Geometry: see drawing. Coordinates: mm, zero at the bounding-box minimum. A direction names the side the tool comes from. Round coordinates to 2 decimals unless told otherwise and drop trailing zeros. Write each loop counter-clockwise with the first axis right and the second up, starting at its lowest first coordinate (ties: lowest second). Pieces come first, ordered by that corner, then holes. Notation, with made-up numbers: (-7.75, 24.5) -> (25.25, 24.5) arc R13 ccw to (25.25, 35.5) -> close; hole circle Ø3 at (77.5, -13). An arc over 180 degrees is marked (long way). Use CSV: the item, a comma, the result in double quotes.
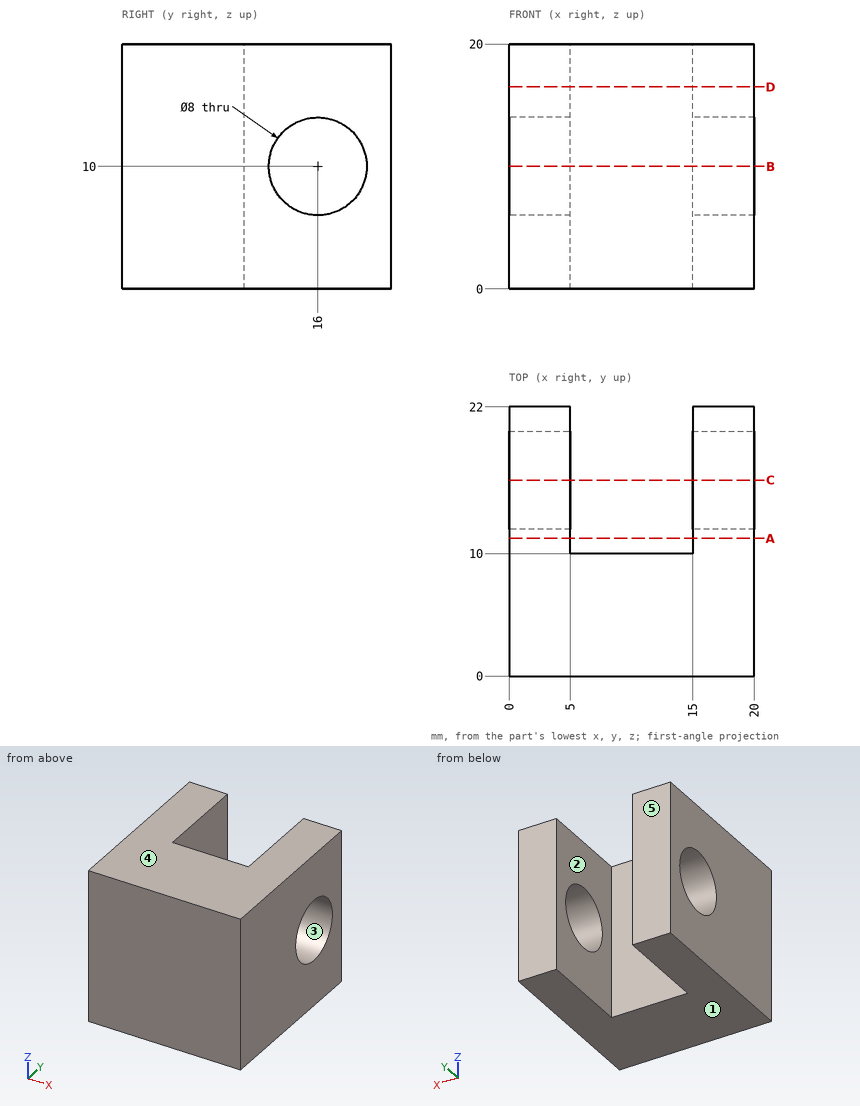
Item 1: Section query A-A on y = 11.25. Return the cut outline in (x, z).
Worked answers:
outline,"(0, 0) -> (5, 0) -> (5, 20) -> (0, 20) -> close; (15, 0) -> (20, 0) -> (20, 20) -> (15, 20) -> close"
Item 2: Set-up query: the marked faces 1 and 2. Return all of +Z, -Z, +X, -X, +Y, -Y with unobstructed straight access to the full face (end or side cutting, diameter ignored); none if empty.
Worked answers:
face 1,"-Z, +X, -X, +Y, -Y"
face 2,"+Z, -Z, +Y"
Item 3: Section query B-B on z = 10. Return the cut outline in (x, y), plus the area to 3 significant figures.
Worked answers:
outline,"(0, 0) -> (20, 0) -> (20, 12) -> (15, 12) -> (15, 10) -> (5, 10) -> (5, 12) -> (0, 12) -> close; (0, 20) -> (5, 20) -> (5, 22) -> (0, 22) -> close; (15, 20) -> (20, 20) -> (20, 22) -> (15, 22) -> close"
area,"240 mm²"
Item 4: Line query: line 1 (Z direction, x = 16.2, y = 16); line 2 (X direction, y = 19, z = 4.25); line 3 (Y direction, x = 16.3, z = 10). Output: solid intervals per line, ascending.
Worked answers:
line 1,"z = 0 to 6, 14 to 20"
line 2,"x = 0 to 5, 15 to 20"
line 3,"y = 0 to 12, 20 to 22"
Item 5: Section query C-C on y = 16. Return the cut outline in (x, z), plus the area to 3 significant figures.
Worked answers:
outline,"(0, 0) -> (5, 0) -> (5, 6) -> (0, 6) -> close; (0, 14) -> (5, 14) -> (5, 20) -> (0, 20) -> close; (15, 0) -> (20, 0) -> (20, 6) -> (15, 6) -> close; (15, 14) -> (20, 14) -> (20, 20) -> (15, 20) -> close"
area,"120 mm²"
Item 6: Pull-direction query (Z, two-part tool) for the marked faces 3, 4 and 5; classes: +Z half, -Z half, draft (parallel to the pull), parting line (faces both ways), or undercut.
Worked answers:
face 3,"undercut"
face 4,"+Z half"
face 5,"draft"
Item 7: First-contact query: pin 1 Ø7 at (y, z) = (16, 10) entering from +X; pin 2 Ø5 at (x, y) = (6.5, 15.5) entering from -Z; pin 3 Ø3 at (x, z) = (11, 12.5) entering from +Y. Flat tips, straight axial feed; report the tip coordinate or a pass-through.
Worked answers:
pin 1,"passes through"
pin 2,"stops at z = 0"
pin 3,"stops at y = 10"
Item 8: Section query D-D on z = 16.5. Return the cut outline in (x, y), plus the area to 3 significant figures.
Worked answers:
outline,"(0, 0) -> (20, 0) -> (20, 22) -> (15, 22) -> (15, 10) -> (5, 10) -> (5, 22) -> (0, 22) -> close"
area,"320 mm²"
